```python
from build123d import *

# Parameters (mm, degrees)
SKETCH1_R           = 10
BOSS_EXTRUDE2_DEPTH = 481.8
BOSS_EXTRUDE4_DEPTH = 75
BOSS_EXTRUDE5_START = -75
BOSS_EXTRUDE5_DEPTH = 75
SKETCH7_R           = 17.483123284
BOSS_EXTRUDE6_DEPTH = 5
BOSS_EXTRUDE7_START = 5
SKETCH8_R           = 17.483123284
BOSS_EXTRUDE7_DEPTH = 5


with BuildPart() as part:
    # Sketch1 → Boss-Extrude2 (new body)
    with BuildSketch(Plane.XY):
        Circle(SKETCH1_R)
    extrude(amount=BOSS_EXTRUDE2_DEPTH)

    # Sketch2 → Boss-Extrude4 (add)
    with BuildSketch(Plane.XY):
        with BuildLine():
            Line((9.029963331, 4.296482543), (17.156826423, 4.296482543))
            Line((17.156826423, 4.296482543), (17.156826423, -3.361979608))
            Line((17.156826423, -3.361979608), (9.417913416, -3.361979608))
            ThreePointArc((9.417913416, -3.361979608), (9.987194288, 0.50591526), (9.029963331, 4.296482543))
        make_face()
        with BuildLine():
            Line((-9.029963331, -4.296482543), (-17.156826423, -4.296482543))
            Line((-17.156826423, -4.296482543), (-17.156826423, 3.361979608))
            Line((-17.156826423, 3.361979608), (-9.417913416, 3.361979608))
            ThreePointArc((-9.417913416, 3.361979608), (-9.987194288, -0.50591526), (-9.029963331, -4.296482543))
        make_face()
    extrude(amount=BOSS_EXTRUDE4_DEPTH)

    # Sketch4 → Boss-Extrude5 (add)
    with BuildSketch(Plane.XY.offset(481.8).offset(BOSS_EXTRUDE5_START)):
        with BuildLine():
            Line((9.029963331, 4.296482543), (17.156826423, 4.296482543))
            Line((17.156826423, 4.296482543), (17.156826423, -3.361979608))
            Line((17.156826423, -3.361979608), (9.417913416, -3.361979608))
            ThreePointArc((9.417913416, -3.361979608), (9.987194288, 0.50591526), (9.029963331, 4.296482543))
        make_face()
        with BuildLine():
            Line((-9.029963331, -4.296482543), (-17.156826423, -4.296482543))
            Line((-17.156826423, -4.296482543), (-17.156826423, 3.361979608))
            Line((-17.156826423, 3.361979608), (-9.417913416, 3.361979608))
            ThreePointArc((-9.417913416, 3.361979608), (-9.987194288, -0.50591526), (-9.029963331, -4.296482543))
        make_face()
    extrude(amount=BOSS_EXTRUDE5_DEPTH)

    # Sketch7 → Boss-Extrude6 (add)
    with BuildSketch(Plane.XY.offset(481.8)):
        with Locations(Location((0, 0, 0), (0, 0, 168.913043394))):
            Circle(SKETCH7_R)
    extrude(amount=BOSS_EXTRUDE6_DEPTH)

    # Sketch8 → Boss-Extrude7 (add)
    with BuildSketch(Plane(origin=(0, 0, 0), x_dir=(-1, 0, 0), z_dir=(0, 0, -1)).offset(BOSS_EXTRUDE7_START)):
        with Locations(Location((0, 0, 0), (0, 0, 11.086956606))):
            Circle(SKETCH8_R)
    extrude(amount=-BOSS_EXTRUDE7_DEPTH)


solid = part.part
```
Verification items for the finished model (mm, model axes). A direction names the side the tool comes from. Give positions to 0.01 mm unless a question says otherwise; leave off trailing zeros. Loops run counter-clockwise (first coordinate to the right, second up) from the corner with the lowest first, then second, coordinate; pieces in that order, holes last. Notation, with made-up numbers: M -28,-19 L -1,-19 A26 ccw -1,6 Z; hole C 7.5,-1.5 d8. An arc over 180 degrees is marked long. One line per question, with ' | ' between items.
Item 1: Thickness scan on line 1 (Z direction, x = -3, y = 15); line 2 (Z direction, x = 10, y = 3.5); line 3 (Y direction, x = -3.5, z = 34.5). Record the ranges inside material, lowest first. Write a range as [from, to].
Completed:
line 1: z = [-5, 0], [481.8, 486.8] | line 2: z = [-5, 75], [406.8, 486.8] | line 3: y = [-9.37, 9.37]
Item 2: Section check B-B, the plane z = 360.5. Record the cut outline in (x, y).
Completed:
outline: C 0,0 d20
Item 3: Depth check by flat-ended pin: P1, Ø1, axis at y = -4, z = 368, coming from the -X side; P2, Ø4, axis at x = 13, z = 429.5, coming from the -Y side; P3, Ø6, axis at y = 2, z = 453.5, coming from the +X side. Enter the tip coordinate at first touch or a pass-through.
Completed:
P1: stops at x = -9.37 | P2: stops at y = -3.36 | P3: stops at x = 17.16
Item 4: Section check A-A, the plane x = 0. Record the cut outline in (y, z).
Completed:
outline: M -17.48,-5 L 17.48,-5 L 17.48,0 L 10,0 L 10,481.8 L 17.48,481.8 L 17.48,486.8 L -17.48,486.8 L -17.48,481.8 L -10,481.8 L -10,0 L -17.48,0 Z
Item 5: Tool access check on faces 1 (the face through (13, 4.296, 37)), 2 (the face through (-2, 11, 481.8)), 3 (the face through (-1, -11, 0)), 4 (the face through (4.614, -8.872, 237.527)). Record the directions out of +Z, -Z, +X, -X, +Y, -Y that give a thin tool (end or side, any length) a straight path to the whole face; none if there is none.
Completed:
face 1: +X, +Y | face 2: +Y | face 3: -Y | face 4: none
